Input: part model. Units: mm. Frame: model coordinates. A direction names the side the tool comes from. Round coordinates to 2 decimals unless told otherwise and drop trailing zeros. Order: outer loops, then holes, each group sorted by start corner. A loop starts at its lowest first (then second) coordinate and runs counter-clockwise, first axis right, second up. Notation, with made-up numbers: (-28, 32) -> (-21, 32) arc R23 ccw to (-21, 71) -> close; hole circle Ø1 at (-6, -0.5). An arc over 180 degrees is marked (long way). Use a Markdown table: item, result.
from build123d import *

# Parameters (mm, degrees)
EXTRUDE_1_DEPTH = 40
EXTRUDE_2_DEPTH = 55
SHELL_1_T       = -6
FILLET_1_R      = 8
FILLET_3_R      = 1


with BuildPart() as part:
    # 스케치1 → 보스-돌출1 (new body)
    with BuildSketch(Plane(origin=(0, 0, 0), x_dir=(1, 0, 0), z_dir=(0, 1, 0))):
        with BuildLine():
            Line((-23.342939481, 38), (30.657060519, 38))
            ThreePointArc((30.657060519, 38), (68.657060519, 0), (30.657060519, -38))
            Line((30.657060519, -38), (-23.342939481, -38))
            ThreePointArc((-23.342939481, -38), (-61.342939481, 0), (-23.342939481, 38))
        make_face()
    extrude(amount=-EXTRUDE_1_DEPTH)

    # 스케치1<3> → 보스-돌출2 (add)
    with BuildSketch(Plane(origin=(0, 0, 0), x_dir=(1, 0, 0), z_dir=(0, 1, 0))):
        with BuildLine():
            Line((-23.342939481, 32), (30.657060519, 32))
            ThreePointArc((30.657060519, 32), (62.657060519, 0), (30.657060519, -32))
            Line((30.657060519, -32), (-23.342939481, -32))
            ThreePointArc((-23.342939481, -32), (-55.342939481, 0), (-23.342939481, 32))
        make_face()
    extrude(amount=-EXTRUDE_2_DEPTH)

    # 쉘1
    shell_1_openings = [part.faces().sort_by_distance(p)[0] for p in [
        (3.657060519, 0, 0),
    ]]
    offset(amount=SHELL_1_T, openings=shell_1_openings, kind=Kind.INTERSECTION)

    # 필렛1
    # the kernel refuses this fillet: 8 mm, written as the material it takes off along each edge
    with BuildSketch(Plane(origin=(30.657060519, -40, 0), x_dir=(0, 0, -1), z_dir=(-1, 0, 0))) as fillet_1_piece_1:
        with BuildLine():
            CenterArc((30, -7.745966692), FILLET_1_R, 0, 75.522487814)
            Line((32, 0), (32.04, 0.154919334))
            ThreePointArc((32.04, 0.154919334), (35, 0.16), (38, 0.16))
            Line((38, 0.16), (38.16, 0))
            Line((38.16, 0), (38.16, -7.745966692))
            Line((38.16, -7.745966692), (38, -7.745966692))
        make_face()
    revolve(axis=Axis((30.657060519, -40, 0), (0, -1, 0)), revolution_arc=180, mode=Mode.SUBTRACT)
    with BuildSketch(Plane(origin=(-23.342939481, -40, -38), x_dir=(0, 0, 1), z_dir=(1, 0, 0))) as fillet_1_piece_2:
        with BuildLine():
            CenterArc((8, -7.745966692), FILLET_1_R, 104.477512186, 75.522487814)
            Line((0, -7.745966692), (-0.16, -7.745966692))
            Line((-0.16, -7.745966692), (-0.16, 0))
            Line((-0.16, 0), (0, 0.16))
            ThreePointArc((0, 0.16), (3, 0.16), (5.96, 0.154919334))
            Line((5.96, 0.154919334), (6, 0))
        make_face()
    extrude(amount=54, mode=Mode.SUBTRACT)
    with BuildSketch(Plane(origin=(30.657060519, -55, 0), x_dir=(0, 0, -1), z_dir=(-1, 0, 0))) as fillet_1_piece_3:
        with BuildLine():
            CenterArc((32 - FILLET_1_R, -FILLET_1_R), FILLET_1_R, 0, 90)
            Line((32 - FILLET_1_R, 0), (32 - FILLET_1_R, FILLET_1_R * 0.02))
            Line((32 - FILLET_1_R, FILLET_1_R * 0.02), (32 + FILLET_1_R * 0.02, FILLET_1_R * 0.02))
            Line((32 + FILLET_1_R * 0.02, FILLET_1_R * 0.02), (32 + FILLET_1_R * 0.02, -FILLET_1_R))
            Line((32 + FILLET_1_R * 0.02, -FILLET_1_R), (32, -FILLET_1_R))
        make_face()
    revolve(axis=Axis((30.657060519, -55, 0), (0, -1, 0)), revolution_arc=180, mode=Mode.SUBTRACT)
    with BuildSketch(Plane(origin=(30.657060519, -55, 32), x_dir=(0, 1, 0), z_dir=(-1, 0, 0)), Plane(origin=(-23.342939481, -55, -32), x_dir=(0, 1, 0), z_dir=(1, 0, 0))) as fillet_1_piece_4:
        with BuildLine():
            CenterArc((FILLET_1_R, FILLET_1_R), FILLET_1_R, 180, 90)
            Line((0, FILLET_1_R), (-FILLET_1_R * 0.02, FILLET_1_R))
            Line((-FILLET_1_R * 0.02, FILLET_1_R), (-FILLET_1_R * 0.02, -FILLET_1_R * 0.02))
            Line((-FILLET_1_R * 0.02, -FILLET_1_R * 0.02), (FILLET_1_R, -FILLET_1_R * 0.02))
            Line((FILLET_1_R, -FILLET_1_R * 0.02), (FILLET_1_R, 0))
        make_face()
    extrude(amount=54, mode=Mode.SUBTRACT)
    with BuildSketch(Plane(origin=(-23.342939481, -55, 0), x_dir=(0, 0, 1), z_dir=(1, 0, 0))) as fillet_1_piece_5:
        with BuildLine():
            CenterArc((32 - FILLET_1_R, -FILLET_1_R), FILLET_1_R, 0, 90)
            Line((32 - FILLET_1_R, 0), (32 - FILLET_1_R, FILLET_1_R * 0.02))
            Line((32 - FILLET_1_R, FILLET_1_R * 0.02), (32 + FILLET_1_R * 0.02, FILLET_1_R * 0.02))
            Line((32 + FILLET_1_R * 0.02, FILLET_1_R * 0.02), (32 + FILLET_1_R * 0.02, -FILLET_1_R))
            Line((32 + FILLET_1_R * 0.02, -FILLET_1_R), (32, -FILLET_1_R))
        make_face()
    revolve(axis=Axis((-23.342939481, -55, 0), (0, -1, 0)), revolution_arc=180, mode=Mode.SUBTRACT)
    with BuildSketch(Plane(origin=(-23.342939481, -40, 0), x_dir=(0, 0, 1), z_dir=(1, 0, 0))) as fillet_1_piece_6:
        with BuildLine():
            CenterArc((30, -7.745966692), FILLET_1_R, 0, 75.522487814)
            Line((32, 0), (32.04, 0.154919334))
            ThreePointArc((32.04, 0.154919334), (35, 0.16), (38, 0.16))
            Line((38, 0.16), (38.16, 0))
            Line((38.16, 0), (38.16, -7.745966692))
            Line((38.16, -7.745966692), (38, -7.745966692))
        make_face()
    revolve(axis=Axis((-23.342939481, -40, 0), (0, -1, 0)), revolution_arc=180, mode=Mode.SUBTRACT)
    with BuildSketch(Plane(origin=(30.657060519, -40, 38), x_dir=(0, 1, 0), z_dir=(-1, 0, 0))) as fillet_1_piece_7:
        with BuildLine():
            CenterArc((7.745966692, 8), FILLET_1_R, 194.477512186, 75.522487814)
            Line((0, 6), (-0.154919334, 5.96))
            ThreePointArc((-0.154919334, 5.96), (-0.16, 3), (-0.16, 0))
            Line((-0.16, 0), (0, -0.16))
            Line((0, -0.16), (7.745966692, -0.16))
            Line((7.745966692, -0.16), (7.745966692, 0))
        make_face()
    extrude(amount=54, mode=Mode.SUBTRACT)

    # 필렛3
    fillet_3_edges = [part.edges().sort_by_distance(p)[0] for p in [
        (3.657060519, -34, -32),
        (-55.342939481, -34, 0),
        (62.657060519, -34, 0),
        (3.657060519, -34, 32),
        (56.657060519, -49, 0),
        (3.657060519, -49, 26),
        (-49.342939481, -49, 0),
        (3.657060519, -49, -26),
    ]]
    fillet(fillet_3_edges, radius=FILLET_3_R)


solid = part.part
1) Cut plane D-D on y = -37.5. Return loops of the section in (x, z), and give its area (3 significant figures).
Results found:
| item | result |
|---|---|
| outline | (-23.34, -36.04) -> (30.66, -36.04) arc R36.04 ccw to (30.66, 36.04) -> (-23.34, 36.04) arc R36.04 ccw to start; hole (-23.34, -26) -> (30.66, -26) arc R26 ccw to (30.66, 26) -> (-23.34, 26) arc R26 ccw to start |
| area | 3,040 mm² |
2) Set-up query: faces 1 (the cylindrical face through (62.65, -43.45, -0.7)), 2 (the cylindrical face through (4.04, -37.21, 36.28)), 3 (the cylindrical face through (-55.335, -43.451, 0.704)), 4 (the flat face through (4, -16, 38)), 5 (the flat face through (4, -49, 0)). Return all of +Z, -Z, +X, -X, +Y, -Y with unobstructed straight access to the full face (end or side cutting, diameter ignored); none if empty.
Results found:
| item | result |
|---|---|
| face 1 | +X, -Y |
| face 2 | +Z, +X, -X, -Y |
| face 3 | -X, -Y |
| face 4 | +Z, +X, -X, +Y, -Y |
| face 5 | +Y |
3) Pull-direction query (Z, two-part tool) for faces 6 (the flat face through (4, 0, 34)), 7 (the cylindrical face through (3.28, -37.21, -36.28)), 8 (the flat face through (3, -16, -32)); classes: +Z half, -Z half, draft (parallel to the pull), parting line (faces both ways), or undercut.
Results found:
| item | result |
|---|---|
| face 6 | draft |
| face 7 | -Z half |
| face 8 | undercut |
4) Line query: L1, parallel to Z at x = 25.5, y = -44; L2, parallel to Z at x = -16, y = -15; L3, parallel to Y at x = 41, z = 6. Output: solid intervals per line, ascending. Write a range as [from, to].
Results found:
| item | result |
|---|---|
| L1 | z = [-32, -26], [26, 32] |
| L2 | z = [-38, -32], [32, 38] |
| L3 | y = [-55, -49] |
5) Cut plane C-C on x = -18.5. Return loops of the section in (y, z), and give its area (3 significant figures).
Results found:
| item | result |
|---|---|
| outline | (-55, -24) arc R8 ccw to (-47, -32) -> (-40, -32) arc R8 ccw to (-32.25, -38) -> (0, -38) -> (0, -32) -> (-33, -32) arc R1 cw to (-34, -31) -> (-34, -26) -> (-48, -26) arc R1 cw to (-49, -25) -> (-49, 25) arc R1 cw to (-48, 26) -> (-34, 26) -> (-34, 31) arc R1 cw to (-33, 32) -> (0, 32) -> (0, 38) -> (-32.25, 38) arc R8 ccw to (-40, 32) -> (-47, 32) arc R8 ccw to (-55, 24) -> close |
| area | 993 mm² |
6) Pin query (flat end, axial travel): pin 1 Ø7.5 at (x, y) = (17, -42) entering from -Z; pin 2 Ø6 at (y, z) = (-27, 21.5) entering from -X; pin 3 Ø15.5 at (x, y) = (3.5, -40.5) entering from +Z. Return the tip coordinate at first contact, or that it passes through.
Results found:
| item | result |
|---|---|
| pin 1 | stops at z = -35.3 |
| pin 2 | stops at x = -56.54 |
| pin 3 | stops at z = 37.98 |
7) Cut plane B-B on y = -16.5. Return loops of the section in (x, z).
Results found:
| item | result |
|---|---|
| outline | (-23.34, -38) -> (30.66, -38) arc R38 ccw to (30.66, 38) -> (-23.34, 38) arc R38 ccw to start; hole (-23.34, -32) -> (30.66, -32) arc R32 ccw to (30.66, 32) -> (-23.34, 32) arc R32 ccw to start |
8) Cut plane A-A on z = 0. Return loops of the section in (x, y), and give its area (3 significant figures).
Results found:
| item | result |
|---|---|
| outline | (-61.34, -32.25) arc R8 ccw to (-55.34, -40) -> (-55.34, -47) arc R8 ccw to (-47.34, -55) -> (54.66, -55) arc R8 ccw to (62.66, -47) -> (62.66, -40) arc R8 ccw to (68.66, -32.25) -> (68.66, 0) -> (62.66, 0) -> (62.66, -33) arc R1 cw to (61.66, -34) -> (56.66, -34) -> (56.66, -48) arc R1 cw to (55.66, -49) -> (-48.34, -49) arc R1 cw to (-49.34, -48) -> (-49.34, -34) -> (-54.34, -34) arc R1 cw to (-55.34, -33) -> (-55.34, 0) -> (-61.34, 0) -> close |
| area | 1,320 mm² |
